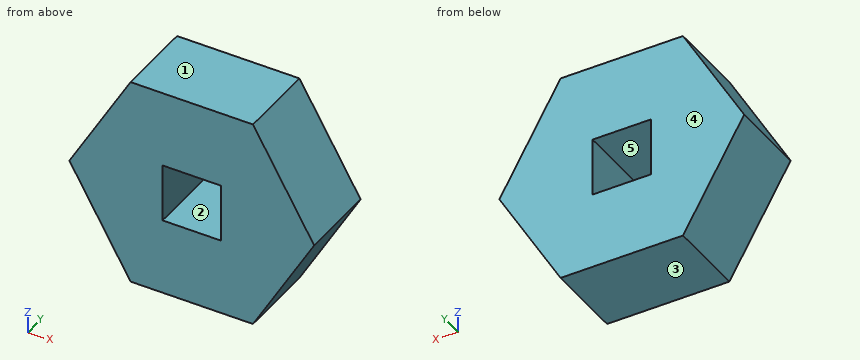
from build123d import *

# Parameters (mm, degrees)
F1_DEPTH = 4.445
F2_W     = 3.302
F2_H     = 3.302
F3_DEPTH = 25.4


with BuildPart() as f1:
    # F0 (on Front) → F1 (new body)
    with BuildSketch(Plane.XZ):
        Polygon((3.460868, 5.9944), (-3.460868, 5.9944), (-6.921737, 0), (-3.460868, -5.9944), (3.460868, -5.9944), (6.921737, 0), align=None)
    extrude(amount=F1_DEPTH)

    # F2 (on face) → F3 (cut)
    with BuildSketch(Plane.XZ.offset(4.445)):
        Rectangle(F2_W, F2_H)
    extrude(amount=-F3_DEPTH, mode=Mode.SUBTRACT)


solid = f1.part
Check sheet for the modelled part. Datum: model origin and axes. Units: mm. Face numbers are marked on the shaded views. A direction names the side the tool comes from. Give positions to 0.01 mm unless a question says otherwise; leave off trailing zeros. Loops run counter-clockwise (first coordinate to the right, second up) from the corner with the lowest first, then second, coordinate; pieces in that order, holes last. Notation, with made-up numbers: M -4.5,-22 L 51.5,-22 A15 ccw 51.5,2 Z; hole C -33,51 d7. An arc over 180 degrees is marked long. Answer as a JSON object with one key per item and string values. Group by question number.
Q1. Cross-section at A-A on y = -0.5. Record the cut outline in (x, z), then the cut area to 3 significant figures.
Q2. Cross-section at D-D on x = 4.25. Record the cut outline in (y, z) (3 decimals).
Q3. Access from +Z, -Z, +X, -X, +Y, -Y to the whole of each face (thin tool, end or side, straight path). Record for the marked faces 1 and 2.
Q4. Cross-section at C-C on x = -0.5. Record the cut outline in (y, z) (3 decimals).
Q5. Material ranges on line 1 along Z through (x, y) = (-1.25, -3.65); line 2 along X through (y, z) = (-1.35, -0.5); line 3 along X through (y, z) = (-3.7, -0.25), recorded low to high. Write a range as [from, to].
Q6. Cross-section at B-B on z = 1.5. Record the cut outline in (x, y) (3 decimals).
Q7. Release check for a two-part mould opening along Z. For the marked faces 3, 4 and 5 record: released by +Z, released by -Z, zero draft, split by the parting line, or undercut.
Q8. Go/stop test with a flat-tipped pin: P1, Ø1, axis at y = -0.5, z = -4, coming from the -X side. Record where the tip stops, or that it passes through.
Evaluation:
{
 "1": {"outline": "M -6.92,0 L -3.46,-5.99 L 3.46,-5.99 L 6.92,0 L 3.46,5.99 L -3.46,5.99 Z; hole M -1.65,-1.65 L 1.65,-1.65 L 1.65,1.65 L -1.65,1.65 Z", "area": "114 mm2"},
 "2": {"outline": "M -4.445,-4.628 L 0,-4.628 L 0,4.628 L -4.445,4.628 Z"},
 "3": {"face 1": "+Z, +X, -X, +Y, -Y", "face 2": "+Y, -Y"},
 "4": {"outline": "M -4.445,-5.994 L 0,-5.994 L 0,-1.651 L -4.445,-1.651 Z; M -4.445,1.651 L 0,1.651 L 0,5.994 L -4.445,5.994 Z"},
 "5": {"line 1": "z = [-5.99, -1.65], [1.65, 5.99]", "line 2": "x = [-6.63, -1.65], [1.65, 6.63]", "line 3": "x = [-6.78, -1.65], [1.65, 6.78]"},
 "6": {"outline": "M -6.056,-4.445 L -1.651,-4.445 L -1.651,0 L -6.056,0 Z; M 1.651,-4.445 L 6.056,-4.445 L 6.056,0 L 1.651,0 Z"},
 "7": {"face 3": "released by -Z", "face 4": "zero draft", "face 5": "undercut"},
 "8": {"P1": "stops at x = -4.9"}
}
